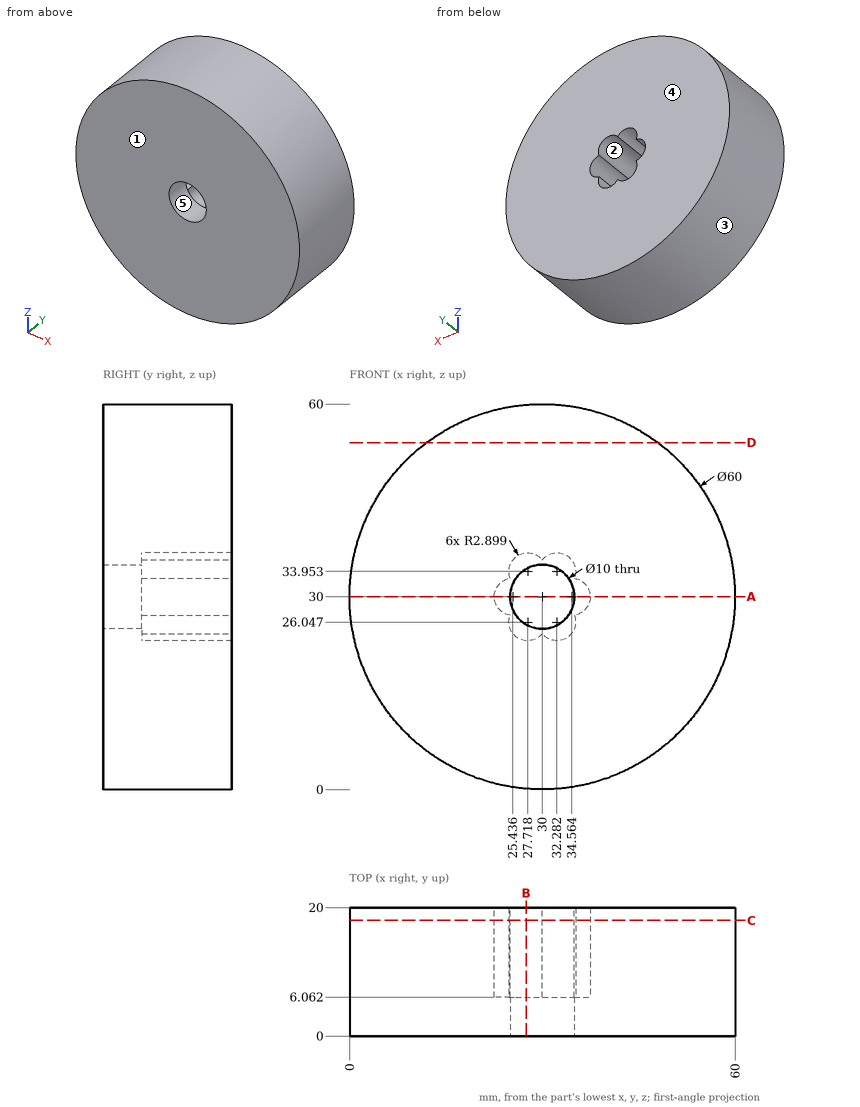
Answer from the drawing. Dimensions are ordinates in mm from the lowest x, y and z of the part. A direction names the side the tool comes from. Coordinates: 2 decimals unless noted, no trailing zeros. Order: outer loops, then holes, each group sorted by start corner. A loop starts at its lowest first (then second) coordinate and runs counter-clockwise, first axis right, second up. Notation, with made-up numbers: (14.5, 71.5) - (49.5, 71.5) arc R15 ccw to (49.5, 97.5) - close; hole circle Ø10 at (-19.5, -25). An arc over 180 degrees is marked (long way). Answer as a JSON object with one key per item and string values. Group by question number.
Item 1: Section D-D (z = 54) is taken. Give the vertices of the cut face in (x, y).
Item 2: Section A-A (z = 30) is taken. Give the vertices of the cut face in (x, y).
Item 3: Section B-B (x = 27.5) is taken. Give the vertices of the cut face in (y, z) (1 decimal).
Item 4: A tool of negligible diameter and unlimited length cuts with its end or side. For the marked faces 1 and 2, from which of +Z, -Z, +X, -X, +Y, -Y can it reach the whole face along a straight path? Write none if from no direction.
Item 5: Consider probe 1 along X at (y, z) = (3.5, 30); probe 2 along X at (y, z) = (19, 35) (1 decimal); probe 3 along Z at (x, y) = (34.5, 17.25). Determine where each line is inside the solid, lowest interval first. Write a range as from..to.
Item 6: The mould has two halves that part along X. Classify the marked faces 3, 4 and 5: +X half, -X half, draft (parallel to the pull), parting line (faces both ways), or undercut.
Item 7: Section C-C (y = 18) is taken. Give the vertices of the cut face in (x, z) (1 decimal), plus the area to 3 significant figures.
Item 8: Flat-ended cylindrical pins translate along their axes: P1, Ø6, axis at x = 17.5, y = 4.5, coming from the +Z side; P2, Ø4, axis at y = 6, z = 8, coming from the +X side; P3, Ø10, axis at x = 47.5, y = 6.5, coming from the -Z side; P4, Ø16, axis at x = 30, z = 30, coming from the -Y side. Find the tip coordinate at first contact, or state that the pin passes through.
Results are:
{
 "1": {"outline": "(12, 0) - (48, 0) - (48, 20) - (12, 20) - close"},
 "2": {"outline": "(0, 0) - (25, 0) - (25, 6.06) - (22.54, 6.06) - (22.54, 20) - (0, 20) - close; (35, 0) - (60, 0) - (60, 20) - (37.46, 20) - (37.46, 6.06) - (35, 6.06) - close"},
 "3": {"outline": "(0, 0.1) - (20, 0.1) - (20, 23.2) - (6.1, 23.2) - (6.1, 25.7) - (0, 25.7) - close; (0, 34.3) - (6.1, 34.3) - (6.1, 36.8) - (20, 36.8) - (20, 59.9) - (0, 59.9) - close"},
 "4": {"face 1": "+Z, -Z, +X, -X, -Y", "face 2": "+Y"},
 "5": {"probe 1": "x = 0..25, 35..60", "probe 2": "x = 0.4..25, 35..59.6", "probe 3": "z = 0.34..24.18, 35.82..59.66"},
 "6": {"face 3": "parting line", "face 4": "draft", "face 5": "undercut"},
 "7": {"outline": "circle Ø60 at (30, 30); hole (25, 27.1) arc R2.9 ccw to (30, 24.3) arc R2.9 ccw to (35, 27.1) arc R2.9 ccw to (35, 32.9) arc R2.9 ccw to (30, 35.7) arc R2.9 ccw to (25, 32.9) arc R2.9 ccw to start", "area": "2,680 mm^2"},
 "8": {"P1": "stops at z = 58.46", "P2": "stops at x = 52.36", "P3": "stops at z = 2.73", "P4": "stops at y = 0"}
}
